from build123d import *

# Parameters (mm, degrees)
SKETCH_1_W           = 123
SKETCH_1_H           = 43
EXTRUDE_1_DEPTH      = 1.5
EXTRUDE_2_DEPTH      = 30
EXTRUDE_2_DEPTH_BACK = 1.5
SKETCH_2_W           = 126
SKETCH_2_H           = 46
SKETCH_2_W_2         = 123
SKETCH_2_H_2         = 43
SKETCH_3_R           = 3.5
EXTRUDE_3_DEPTH      = 5
SKETCH_5_R           = 1.6
CUT_EXTRUDE_1_DEPTH  = 10
CUT_EXTRUDE_2_DEPTH  = 10
SKETCH_7_W           = 14.5
SKETCH_7_H           = 9
CUT_EXTRUDE_3_DEPTH  = 10
FILLET_1_R           = 2


with BuildPart() as part:
    # Эскиз1 → Бобышка-Вытянуть1 (new body)
    with BuildSketch(Plane.XY):
        with Locations((61.5, 21.5)):
            Rectangle(SKETCH_1_W, SKETCH_1_H)
    extrude(amount=EXTRUDE_1_DEPTH)

    # Эскиз2 → Бобышка-Вытянуть2 (add, two sides: drawn at the far end of the back side and taken through both)
    with BuildSketch(Plane(origin=(0, 0, 0), x_dir=(-1, 0, 0), z_dir=(0, 0, -1)).offset(-EXTRUDE_2_DEPTH_BACK)):
        with Locations((-61.5, 21.5)):
            Rectangle(SKETCH_2_W, SKETCH_2_H)
        with Locations((-61.5, 21.5)):
            Rectangle(SKETCH_2_W_2, SKETCH_2_H_2, mode=Mode.SUBTRACT)
    extrude(amount=EXTRUDE_2_DEPTH + EXTRUDE_2_DEPTH_BACK)

    # Эскиз3 → Бобышка-Вытянуть3 (add)
    with BuildSketch(Plane(origin=(0, 0, -30), x_dir=(-1, 0, 0), z_dir=(0, 0, -1))):
        with BuildLine():
            Line((-124.5, 12.5), (-132.54002612, 12.5))
            ThreePointArc((-132.54002612, 12.5), (-141.54002612, 21.5), (-132.54002612, 30.5))
            Line((-132.54002612, 30.5), (-124.5, 30.5))
            Line((-124.5, 30.5), (-124.5, 12.5))
        make_face()
        with Locations((-132.54002612, 21.5)):
            Circle(SKETCH_3_R, mode=Mode.SUBTRACT)
    extrude_3 = extrude(amount=-EXTRUDE_3_DEPTH)

    # Зеркальное отражение1: Бобышка-Вытянуть3 across plane
    add(extrude_3.mirror(Plane(origin=(61.5, 0, 0), x_dir=(0, 0, 1), z_dir=(1, 0, 0))))

    # Эскиз5 → Вырез-Вытянуть1 (cut)
    with BuildSketch(Plane.XY.offset(1.5)):
        with Locations((69.5, 4.7)):
            Circle(SKETCH_5_R)
    extrude(amount=-CUT_EXTRUDE_1_DEPTH, mode=Mode.SUBTRACT)

    # Эскиз6 → Вырез-Вытянуть2 (cut)
    with BuildSketch(Plane.ZY.offset(1.5)):
        Polygon((-20, 17.3), (-22.5, 17.3), (-25, 17.3), (-25, 16.65), (-25, 9.65), (-25, 8.5), (-22.5, 8.5), (-20, 8.5), align=None)
    extrude(amount=-CUT_EXTRUDE_2_DEPTH, mode=Mode.SUBTRACT)

    # Эскиз7 → Вырез-Вытянуть3 (cut)
    with BuildSketch(Plane(origin=(0, 44.5, 0), x_dir=(1, 0, 0), z_dir=(0, 1, 0))):
        with Locations((55.75, 8)):
            Rectangle(SKETCH_7_W, SKETCH_7_H)
    extrude(amount=-CUT_EXTRUDE_3_DEPTH, mode=Mode.SUBTRACT)

    # Скругление1
    fillet_1_edges = [part.edges().sort_by_distance(p)[0] for p in [
        (124.5, 30.5, -27.5),
        (124.5, 12.5, -27.5),
        (-1.5, 12.5, -27.5),
        (-1.5, 30.5, -27.5),
    ]]
    fillet(fillet_1_edges, radius=FILLET_1_R)


solid = part.part
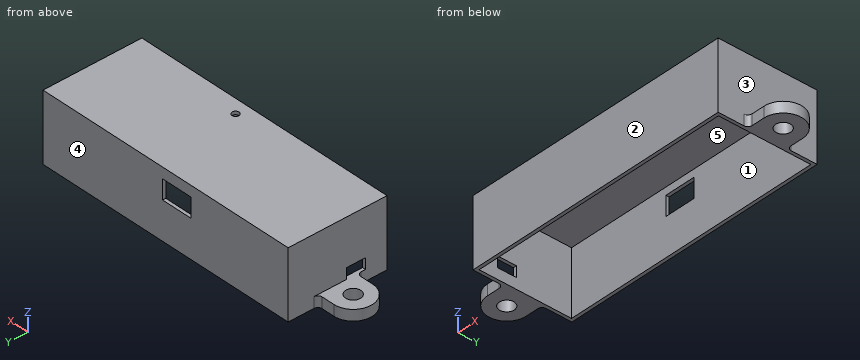
CAD build for the part. Positions are in the model's coordinates, mm. Face numbers are marked on the shaded views. A direction names the side the tool comes from. Round coordinates to 2 decimals unless told otherwise and drop trailing zeros. Write each loop counter-clockwise with the first axis right and the second up, starting at its lowest first coordinate (ties: lowest second). Pieces come first, ordered by that corner, then holes. Notation, with made-up numbers: M -19.75,10 L 15.25,10 A18 ccw 15.25,32 Z; hole C 47.5,47.5 d6. An arc over 180 degrees is marked long. Use a Markdown table: item, result. Add a question column.
1. Slice it at D-D on y = 4.7. Give the cut face in (x, z), then the cut area to 3 significant figures.
2. Pull direction X, two halves, no side cores. Call the marked faces 1, 2 and 3: released by +X, released by -X, zero draft, split by the parting line, or undercut.
3. Slice it at C-C on z = -8. Give the cut face in (x, y).
4. Slice it at B-B on y = 21.5. Give the cut face in (x, z), then the cut area to 3 significant figures.
5. Drill centre lines: probe 1 along Y at (x, z) = (102.5, -19.5); probe 2 along X at (y, z) = (29, -10.5); probe 3 along X at (y, z) = (19, -26.5). Where is each one in solid material? Low to high.
6. Flat gauge pins, fed straight in: P1, Ø21.5, axis at x = 41.5, y = 14, coming from the -Z side; P2, Ø5.5, axis at x = 129.5, z = -26.5, coming from the +Y side; P3, Ø8.5, axis at x = 137, y = 21, coming from the +Z side. Where does each tip first touch, or does it go through?
7. Slice it at A-A on x = 69.5. Give the cut face in (y, z), then the cut area to 3 significant figures.
8. 3-axis set-ups, long thin cutter, end or side, ignore diameter. For the marked faces 4 and 5: which of +Z, -Z, +X, -X, +Y, -Y reach the whole face in a straight line?
Reply:
| question | item | result |
|---|---|---|
| 1 | outline | M -1.5,-30 L 0,-30 L 0,0 L 67.9,0 L 67.9,1.5 L -1.5,1.5 Z; M 71.1,0 L 123,0 L 123,-30 L 124.5,-30 L 124.5,1.5 L 71.1,1.5 Z |
| 1 | area | 274 mm^2 |
| 2 | face 1 | undercut |
| 2 | face 2 | zero draft |
| 2 | face 3 | released by +X |
| 3 | outline | M -1.5,-1.5 L 124.5,-1.5 L 124.5,44.5 L 63,44.5 L 63,43 L 123,43 L 123,0 L 0,0 L 0,43 L 48.5,43 L 48.5,44.5 L -1.5,44.5 Z |
| 4 | outline | M -18.54,-30 L -13.04,-30 L -13.04,-25 L -18.54,-25 Z; M -6.04,-30 L 0,-30 L 0,0 L 123,0 L 123,-30 L 129.04,-30 L 129.04,-25 L 124.5,-25 L 124.5,1.5 L -1.5,1.5 L -1.5,-25 L -6.04,-25 Z; M 136.04,-30 L 141.54,-30 L 141.54,-25 L 136.04,-25 Z |
| 4 | area | 379 mm^2 |
| 5 | probe 1 | y = -1.5 to 0, 43 to 44.5 |
| 5 | probe 2 | x = -1.5 to 0, 123 to 124.5 |
| 5 | probe 3 | x = -18.19 to -11.99, -7.09 to 0, 123 to 130.09, 134.99 to 141.19 |
| 6 | P1 | stops at z = 0 |
| 6 | P2 | stops at y = 30.5 |
| 6 | P3 | stops at z = -25 |
| 7 | outline | M -1.5,-30 L 0,-30 L 0,0 L 3.1,0 L 3.1,1.5 L -1.5,1.5 Z; M 6.3,0 L 43,0 L 43,-30 L 44.5,-30 L 44.5,1.5 L 6.3,1.5 Z |
| 7 | area | 154 mm^2 |
| 8 | face 4 | +Z, -Z, +X, -X, +Y |
| 8 | face 5 | -Z |
